The model under review builds one solid part; all positions refer to its coordinate system, in mm. Face numbers are marked on the shaded views. A direction names the side the tool comes from. Give positions to 0.01 mm unless a question says otherwise; leave off trailing zeros. Order: outer loops, then holes, each group sorted by start corner. A loop starts at its lowest first (then second) coordinate and runs counter-clockwise, first axis right, second up.
```python
from build123d import *

# Parameters (mm, degrees)
F0_W     = 254
F0_H     = 177.8
F0_R     = 1.905
F0_R_2   = 5.08
F0_R_3   = 3.175
F0_R_4   = 5.715
F0_W_2   = 44.45
F0_H_2   = 31.75
F0_W_3   = 98.2218
F0_H_3   = 39.8018
F1_DEPTH = 25.4


with BuildPart() as f1:
    # F0 (on Front) → F1 (new body)
    with BuildSketch(Plane.XZ):
        with Locations((127, -88.9)):
            Rectangle(F0_W, F0_H)
        with Locations((64.135, -130.175)):
            Circle(F0_R, mode=Mode.SUBTRACT)
        with Locations((168.275, -158.75)):
            Circle(F0_R_2, mode=Mode.SUBTRACT)
        with Locations((200.025, -158.75)):
            Circle(F0_R_2, mode=Mode.SUBTRACT)
        with Locations((152.4, -120.65)):
            Circle(F0_R_3, mode=Mode.SUBTRACT)
        with Locations((184.15, -133.35)):
            Circle(F0_R_2, mode=Mode.SUBTRACT)
        with Locations((215.9, -133.35)):
            Circle(F0_R_2, mode=Mode.SUBTRACT)
        with Locations((238.76, -123.825)):
            Circle(F0_R_4, mode=Mode.SUBTRACT)
        with Locations((64.135, -88.9)):
            Rectangle(F0_W_2, F0_H_2, mode=Mode.SUBTRACT)
        with Locations((64.135, -47.625)):
            Circle(F0_R, mode=Mode.SUBTRACT)
        with Locations((140.5382, -67.31)):
            Circle(F0_R, mode=Mode.SUBTRACT)
        with Locations((158.75, -88.9)):
            Circle(F0_R_2, mode=Mode.SUBTRACT)
        with Locations((200.025, -82.55)):
            Circle(F0_R_3, mode=Mode.SUBTRACT)
        with Locations((241.3, -82.55)):
            Circle(F0_R_3, mode=Mode.SUBTRACT)
        with Locations((233.68, -67.31)):
            Circle(F0_R, mode=Mode.SUBTRACT)
        with Locations((187.1091, -39.7891)):
            Rectangle(F0_W_3, F0_H_3, mode=Mode.SUBTRACT)
        with Locations((140.5382, -12.2682)):
            Circle(F0_R, mode=Mode.SUBTRACT)
        with Locations((233.68, -12.2682)):
            Circle(F0_R, mode=Mode.SUBTRACT)
    extrude(amount=F1_DEPTH)


solid = f1.part
```
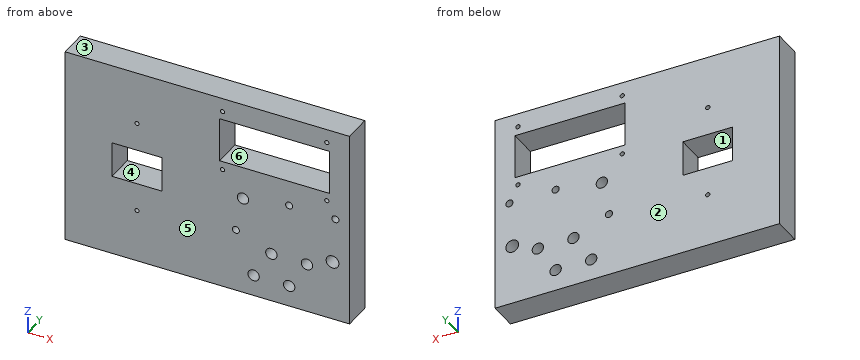
1. Draft analysis for pull direction Z (two halves, no side actions). For the marked faces 3, 4, 5 and 6, state which applies: pulls with the +Z half, pulls with the -Z half, needs draft (parallel to the pull), parting line crosses it, or undercut.
2. Take a section at C-C (y = -21). Count the separate pieces of the cut face and the enclosed holes in it, and give its area (3 significant figures).
3. Take a section at D-D (z = -120.65). Write out the cut boundary in (x, y) (3 decimals).
4. Take a section at A-A (z = -53). Write out the cut boundary in (x, y), and give its area (3 significant figures).
5. To check wall thickness, follow line 1 (Z direction, x = 141, y = -14); line 2 (X direction, y = -19.5, z = -67.31) (3 decimals); line 3 (X direction, y = -18, z = -133). State the ranges of each line that lie inside material, in increasing order.
6. For the marked faces 1 and 2, list the 3-axis set-ups (+Z, -Z, +X, -X, +Y, -Y) from which the entire face can be reached by the end or side of a thin tool; tool diameter is ignored.
7. Take a section at B-B (x = 145). Write out the cut boundary in (y, z).
Answer:
1. face 3: pulls with the +Z half
1. face 4: undercut
1. face 5: needs draft
1. face 6: undercut
2. separate pieces: 1
2. enclosed holes: 17
2. area: 39,200 mm2
3. outline: (0, -25.4) - (149.225, -25.4) - (149.225, 0) - (0, 0) - close; (155.575, -25.4) - (234.008, -25.4) - (234.008, 0) - (155.575, 0) - close; (243.512, -25.4) - (254, -25.4) - (254, 0) - (243.512, 0) - close
4. outline: (0, -25.4) - (138, -25.4) - (138, 0) - (0, 0) - close; (236.22, -25.4) - (254, -25.4) - (254, 0) - (236.22, 0) - close
4. area: 3,960 mm2
5. line 1: z = -177.8 to -69.16, -65.46 to -59.69, -19.89 to -14.12, -10.42 to 0
5. line 2: x = 0 to 138.633, 142.443 to 231.775, 235.585 to 254
5. line 3: x = 0 to 179.08, 189.22 to 210.83, 220.97 to 254
6. face 1: +Y, -Y
6. face 2: +Z, -Z, +X, -X, +Y
7. outline: (-25.4, -177.8) - (0, -177.8) - (0, -59.69) - (-25.4, -59.69) - close; (-25.4, -19.89) - (0, -19.89) - (0, 0) - (-25.4, 0) - close
